```python
from build123d import *

# Parameters (mm, degrees)
SKETCH_1_W               = 20
SKETCH_1_H               = 10
EXTRUDE_1_DEPTH          = 9
CUT_EXTRUDE_3_DEPTH      = 9
CUT_EXTRUDE_4_DEPTH      = 18.52868966
CUT_EXTRUDE_4_DEPTH_BACK = 9
EXTRUDE_2_DEPTH          = 9
EXTRUDE_3_DEPTH          = 9
SKETCH_10_W              = 8
SKETCH_10_H              = 13
CUT_EXTRUDE_5_DEPTH      = 9
SKETCH_12_W              = 2.5
SKETCH_12_H              = 12
CUT_EXTRUDE_6_DEPTH      = 9
SKETCH_13_W              = 2.5
SKETCH_13_H              = 7.75
CUT_EXTRUDE_7_DEPTH      = 9
CUT_EXTRUDE_8_DEPTH      = 9
CUT_EXTRUDE_9_DEPTH      = 9
SKETCH_26_R              = 0.25
CUT_EXTRUDE_16_DEPTH     = 19.638541659
SCALE_1_SCALE            = 2.454545455
SKETCH_29_W              = 19.36913475
SKETCH_29_H              = 8.233667945
CUT_EXTRUDE_17_DEPTH     = 35.391743647
CUT_EXTRUDE_18_DEPTH     = 10
SKETCH_34_R              = 0.615
CUT_EXTRUDE_19_DEPTH     = 10
CUT_EXTRUDE_20_DEPTH     = 10


with BuildPart() as part:
    # 草图1 → 凸台-拉伸1 (new body)
    with BuildSketch(Plane(origin=(0, 0, 0), x_dir=(0, 0, -1), z_dir=(1, 0, 0))):
        with Locations((-3.964524465, 0.58990319)):
            Rectangle(SKETCH_1_W, SKETCH_1_H)
    extrude(amount=EXTRUDE_1_DEPTH)

    # 草图2 → 切除-拉伸3 (cut)
    with BuildSketch(Plane(origin=(9, 0, 0), x_dir=(0, 0, -1), z_dir=(1, 0, 0))):
        Polygon((0.035475535, -0.41009681), (-3.964524465, -4.41009681), (6.035475535, -4.41009681), (6.035475535, -0.410096535), align=None)
    extrude(amount=-CUT_EXTRUDE_3_DEPTH, mode=Mode.SUBTRACT)

    # 草图6 → 切除-拉伸4 (cut, two sides: drawn at the far end of the back side and taken through both)
    with BuildSketch(Plane(origin=(9, 0, 0), x_dir=(0, 0, -1), z_dir=(1, 0, 0)).offset(-CUT_EXTRUDE_4_DEPTH_BACK)):
        Polygon((-66.684543288, -0.910096672), (-13.964524465, -0.910096672), (-3.964524465, -0.910096672), (0.035475535, 3.089903328), (6.035475535, 3.089903328), (58.755494358, 3.089903328), (55.394957379, 108.476374614), (-70.045080267, 104.476374614), align=None)
    extrude(amount=CUT_EXTRUDE_4_DEPTH + CUT_EXTRUDE_4_DEPTH_BACK, mode=Mode.SUBTRACT)

    # 草图8 → 凸台-拉伸2 (add)
    with BuildSketch(Plane(origin=(9, 0, 0), x_dir=(0, 0, -1), z_dir=(1, 0, 0))):
        with BuildLine():
            Line((-13.964524465, -4.41009681), (-13.964524465, -0.910096672))
            ThreePointArc((-13.964524465, -0.910096672), (-15.714524534, -2.660096741), (-13.964524465, -4.41009681))
        make_face()
    extrude(amount=-EXTRUDE_2_DEPTH)

    # 草图9 → 凸台-拉伸3 (add)
    with BuildSketch(Plane(origin=(9, 0, 0), x_dir=(0, 0, -1), z_dir=(1, 0, 0))):
        with BuildLine():
            Line((6.035475535, -0.410096672), (6.035475535, 3.089903328))
            ThreePointArc((6.035475535, 3.089903328), (7.785475535, 1.339903328), (6.035475535, -0.410096672))
        make_face()
    extrude(amount=-EXTRUDE_3_DEPTH)

    # 草图10 → 切除-拉伸5 (cut)
    with BuildSketch(Plane(origin=(0, -0.910096672, 0), x_dir=(1, 0, 0), z_dir=(0, 1, 0))):
        with Locations((4.5, -10.464524465)):
            Rectangle(SKETCH_10_W, SKETCH_10_H)
    extrude(amount=-CUT_EXTRUDE_5_DEPTH, mode=Mode.SUBTRACT)

    # 草图12 → 切除-拉伸6 (cut)
    with BuildSketch(Plane(origin=(0, 3.089903328, 0), x_dir=(1, 0, 0), z_dir=(0, 1, 0))):
        with Locations((7.75, 6.035475535)):
            Rectangle(SKETCH_12_W, SKETCH_12_H)
    extrude(amount=-CUT_EXTRUDE_6_DEPTH, mode=Mode.SUBTRACT)

    # 草图13 → 切除-拉伸7 (cut)
    with BuildSketch(Plane(origin=(0, 3.089903328, 0), x_dir=(1, 0, 0), z_dir=(0, 1, 0))):
        with Locations((1.25, 3.910475535)):
            Rectangle(SKETCH_13_W, SKETCH_13_H)
    extrude(amount=-CUT_EXTRUDE_7_DEPTH, mode=Mode.SUBTRACT)

    # 草图14 → 切除-拉伸8 (cut)
    with BuildSketch(Plane(origin=(0, 1.527213896, 1.527213896), x_dir=(1, 0, 0), z_dir=(0, 0.7071067811865477, 0.7071067811865475))):
        Polygon((2.5, 2.209976588), (0, -3.446877662), (-6.872938914, -0.617067375), (-4.372938914, 5.039786874), align=None)
    extrude(amount=-CUT_EXTRUDE_8_DEPTH, mode=Mode.SUBTRACT)

    # 草图15 → 切除-拉伸9 (cut)
    with BuildSketch(Plane(origin=(0, 1.527213896, 1.527213896), x_dir=(1, 0, 0), z_dir=(0, 0.7071067811865477, 0.7071067811865475))):
        Polygon((6.5, 2.209976588), (9, -3.446877662), (12.673354488, 0), (10.173354488, 5.656854249), align=None)
    extrude(amount=-CUT_EXTRUDE_9_DEPTH, mode=Mode.SUBTRACT)

    # 草图26 → 切除-拉伸16 (cut, through all)
    with BuildSketch(Plane.ZY):
        with Locations((13.964524465, -2.660096741)):
            Circle(SKETCH_26_R)
    extrude(amount=-CUT_EXTRUDE_16_DEPTH, mode=Mode.SUBTRACT)


with BuildPart() as part_1:
    # 缩放比例1: scaled about (4.5, -0.253377538, 0.893630972)
    add(part.part.scale(SCALE_1_SCALE).moved(Location((-6.545454545, 0.368549146, -1.299826868))))

    # 草图29 → 切除-拉伸17 (cut, through all)
    with BuildSketch(Plane.XY.offset(8.431278652)):
        with Locations((4.462607848, 10.069691287)):
            Rectangle(SKETCH_29_W, SKETCH_29_H)
    extrude(amount=-CUT_EXTRUDE_17_DEPTH, mode=Mode.SUBTRACT)

    # 草图31 → 切除-拉伸18 (cut)
    with BuildSketch(Plane(origin=(9.409090909, 0, 0), x_dir=(0, 0, -1), z_dir=(1, 0, 0))):
        with BuildLine():
            Line((19.210193521, 0.679886253), (1.386903166, 0.679886253))
            Line((1.386903166, 0.679886253), (1.386903166, -0.638052115))
            Line((1.386903166, -0.638052115), (16.114175893, -0.638051777))
            ThreePointArc((16.114175893, -0.638051777), (17.796606115, -0.29485713), (19.210193521, 0.679886253))
        make_face()
    extrude(amount=-CUT_EXTRUDE_18_DEPTH, mode=Mode.SUBTRACT)

    # 草图34 → 切除-拉伸19 (cut)
    with BuildSketch(Plane(origin=(9.409090909, 0, 0), x_dir=(0, 0, -1), z_dir=(1, 0, 0))):
        with Locations((15.522596163, 3.658191587)):
            Circle(SKETCH_34_R)
    extrude(amount=-CUT_EXTRUDE_19_DEPTH, mode=Mode.SUBTRACT)

    # 草图35 → 切除-拉伸20 (cut)
    with BuildSketch(Plane(origin=(9.409090909, 0, 0), x_dir=(0, 0, -1), z_dir=(1, 0, 0))):
        Polygon((18.603278237, 9.002231919), (19.169117802, -10.424926464), (26.96512958, -9.984829025), (26.399290016, 9.442329358), align=None)
    extrude(amount=-CUT_EXTRUDE_20_DEPTH, mode=Mode.SUBTRACT)


solid = part_1.part
```
Could you check a few things on this model? Use its own coordinates, in mm. A direction names the side the tool comes from. Give positions to 0.01 mm unless a question says otherwise; leave off trailing zeros. Order: outer loops, then holes, each group sorted by start corner. A loop starts at its lowest first (then second) coordinate and runs counter-clockwise, first axis right, second up.
Q1. Suppose I cut it at D-D, the plane z = 5.5. Write out the boundary of the cut face in (x, y), and give its area (3 significant figures).
Q2. We'd pull the mould along X, two halves only. Please class faces 1 (the flat face through (14.318, -6, 23)), 2 (the flat face through (-6.545, -6, 20)), 3 (the flat face through (-6, -1.865, 21)): +X half, -X half, draft (parallel to the pull), parting line (faces both ways), or undercut.
Q3. For faces 4 (the flat face through (15, -1.865, 21)), 5 (the flat face through (9.409, 3, -10)), 6 (the flat face through (-5.318, -6, 23)), 7 (the flat face through (-0.409, 3, -10)), 8 (the flat face through (15.545, -6, 20)), which set-ups out of +Z, -Z, +X, -X, +Y, -Y let a thin tool reach every point of the face, with its end or its side?
Q4. Suppose I cut it at C-C, the plane y = -3.5. Write out the boundary of the cut face in (x, z), and give its area (3 significant figures).
Q5. Suppose I cut it at B-B, the plane x = 7. Write out the boundary of the cut face in (y, z) (3 decimals).
Q6. If I drill on line 1 along X through (y, z) = (-9.5, 25); line 2 along Y through (x, z) = (6.5, -7.5); line 3 along X through (y, z) = (1.25, -13), over which ranges is the centre line in solid material (lowest first)?
Q7. Suppose I cut it at A-A, the plane z = 22. Write out the boundary of the cut face in (x, y).
Q8. I'm going to push flat-ended pins straight in: P1, Ø1, axis at x = -6, z = 24.5, coming from the +Y side; P2, Ø0.7, axis at y = -6.16, z = 32.98, coming from the +X side; P3, Ø9.5, axis at x = 6, y = -6.5, coming from the +Z side; P4, Ø6, axis at y = 2.5, z = -7.5, coming from the -X side. Where does each tip first touch, or does it pass through?
Solution:
1. outline: (-6.55, -7.52) - (15.55, -7.52) - (15.55, -4.8) - (13.71, 1.07) - (-4.71, 1.07) - (-6.55, -4.8) - close
1. area: 179 mm2
2. face 1: undercut
2. face 2: -X half
2. face 3: draft
3. face 4: +Z, +X, -X, +Y
3. face 5: -Z, +X, +Y, -Y
3. face 6: +Z, +Y, -Y
3. face 7: -Z, -X, +Y, -Y
3. face 8: +Z, -Z, +X, +Y, -Y
4. outline: (-6.55, 6.8) - (-4.88, 1.48) - (13.88, 1.48) - (15.55, 6.8) - (15.55, 36.35) - (14.32, 36.35) - (14.32, 8.43) - (-5.32, 8.43) - (-5.32, 36.35) - (-6.55, 36.35) - close
4. area: 213 mm2
5. outline: (-10.456, 8.431) - (-0.638, -1.387) - (0.68, -1.387) - (0.68, -18.846) - (5.953, -18.692) - (5.953, 0.613) - (-1.865, 8.431) - close; hole circle Ø1.23 at (3.658, -15.523)
6. line 1: x = -6.55 to -5.32, 14.32 to 15.55
6. line 2: y = 0.68 to 5.95
6. line 3: x = -0.41 to 9.41
7. outline: (-6.55, -10.46) - (-5.32, -10.46) - (-5.32, -1.87) - (-6.55, -1.87) - close; (14.32, -10.46) - (15.55, -10.46) - (15.55, -1.87) - (14.32, -1.87) - close
8. P1: stops at y = -1.87
8. P2: passes through
8. P3: stops at z = 8.43
8. P4: stops at x = -0.41
